Design review of the part built by this model. Coordinates are the model's own, in mm. Face numbers are marked on the shaded views. A direction names the side the tool comes from. Round coordinates to 2 decimals unless told otherwise and drop trailing zeros. Order: outer loops, then holes, each group sorted by start corner. A loop starts at its lowest first (then second) coordinate and runs counter-clockwise, first axis right, second up. Notation, with made-up numbers: (-26, -26.75) - (32, -26.75) arc R22 cw to (32, -7.75) - close; hole circle Ø11 at (21, -27.75). An arc over 180 degrees is marked (long way). Write item = value, one per line.
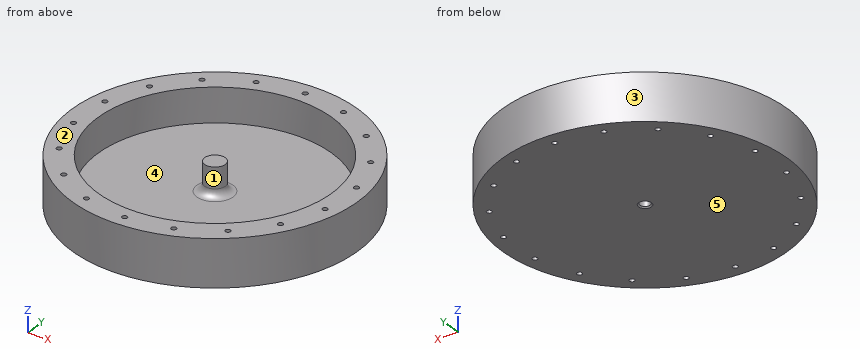
from build123d import *

# Parameters (mm, degrees)
SKETCH1_R                = 4
SKETCH1_R_2              = 2
BOSS_EXTRUDE1_DEPTH      = 8
BOSS_EXTRUDE2_START      = -8
SKETCH2_R                = 45
SKETCH2_R_2              = 4
BOSS_EXTRUDE2_DEPTH      = 5
BOSS_EXTRUDE3_START      = -8
SKETCH3_R                = 55
SKETCH3_R_2              = 45
BOSS_EXTRUDE3_DEPTH      = 18.1
SKETCH4_R                = 2
BOSS_EXTRUDE4_DEPTH      = 2
SKETCH5_R                = 1
CUT_EXTRUDE1_DEPTH       = 5
CIRPATTERN1_COUNT        = 18
MIRROR1_COPY_1_SKETCH_R  = 1
MIRROR1_COPY_1_DEPTH     = 5
MIRROR1_COPY_2_SKETCH_R  = 1
MIRROR1_COPY_2_DEPTH     = 5
MIRROR1_COPY_3_SKETCH_R  = 1
MIRROR1_COPY_3_DEPTH     = 5
MIRROR1_COPY_4_SKETCH_R  = 1
MIRROR1_COPY_4_DEPTH     = 5
MIRROR1_COPY_5_SKETCH_R  = 1
MIRROR1_COPY_5_DEPTH     = 5
MIRROR1_COPY_6_SKETCH_R  = 1
MIRROR1_COPY_6_DEPTH     = 5
MIRROR1_COPY_7_SKETCH_R  = 1
MIRROR1_COPY_7_DEPTH     = 5
MIRROR1_COPY_8_SKETCH_R  = 1
MIRROR1_COPY_8_DEPTH     = 5
MIRROR1_COPY_9_SKETCH_R  = 1
MIRROR1_COPY_9_DEPTH     = 5
MIRROR1_COPY_10_SKETCH_R = 1
MIRROR1_COPY_10_DEPTH    = 5
MIRROR1_COPY_11_SKETCH_R = 1
MIRROR1_COPY_11_DEPTH    = 5
MIRROR1_COPY_12_SKETCH_R = 1
MIRROR1_COPY_12_DEPTH    = 5
MIRROR1_COPY_13_SKETCH_R = 1
MIRROR1_COPY_13_DEPTH    = 5
MIRROR1_COPY_14_SKETCH_R = 1
MIRROR1_COPY_14_DEPTH    = 5
MIRROR1_COPY_15_SKETCH_R = 1
MIRROR1_COPY_15_DEPTH    = 5
MIRROR1_COPY_16_SKETCH_R = 1
MIRROR1_COPY_16_DEPTH    = 5
MIRROR1_COPY_17_SKETCH_R = 1
MIRROR1_COPY_17_DEPTH    = 5
CHAMFER1_SIZE            = 0.5
FILLET1_R                = 3


with BuildPart() as part:
    # Sketch1 → Boss-Extrude1 (new body, symmetric)
    with BuildSketch(Plane.XY):
        Circle(SKETCH1_R)
        Circle(SKETCH1_R_2, mode=Mode.SUBTRACT)
    extrude(amount=BOSS_EXTRUDE1_DEPTH, both=True)

    # Sketch2 → Boss-Extrude2 (add)
    with BuildSketch(Plane.XY.offset(BOSS_EXTRUDE2_START)):
        Circle(SKETCH2_R)
        Circle(SKETCH2_R_2, mode=Mode.SUBTRACT)
    extrude(amount=BOSS_EXTRUDE2_DEPTH)

    # Sketch3 → Boss-Extrude3 (add)
    with BuildSketch(Plane.XY.offset(BOSS_EXTRUDE3_START)):
        Circle(SKETCH3_R)
        Circle(SKETCH3_R_2, mode=Mode.SUBTRACT)
    extrude(amount=BOSS_EXTRUDE3_DEPTH)

    # Sketch4 → Boss-Extrude4 (add)
    with BuildSketch(Plane.XY.offset(8)):
        Circle(SKETCH4_R)
    extrude(amount=-BOSS_EXTRUDE4_DEPTH)

    # Sketch5 → Cut-Extrude1 (cut)
    with BuildSketch(Plane.XY.offset(10.1)):
        with Locations((0, 50)):
            Circle(SKETCH5_R)
    cut_extrude1 = extrude(amount=-CUT_EXTRUDE1_DEPTH, mode=Mode.SUBTRACT)

    # CirPattern1: Cut-Extrude1 ×18 about axis
    cirpattern1_axis = Axis((0, 0, 0), (0, 0, 1))
    for i in range(1, CIRPATTERN1_COUNT):
        add(cut_extrude1.rotate(cirpattern1_axis, i * 360 / CIRPATTERN1_COUNT), mode=Mode.SUBTRACT)

    # Mirror1: Cut-Extrude1 across plane
    add(cut_extrude1.mirror(Plane.XY.offset(1.05)), mode=Mode.SUBTRACT)

    # Mirror1 copy 1 sketch → Mirror1 copy 1 (cut)
    with BuildSketch(Plane(origin=(0, 0, -8), x_dir=(0.939692621, 0.342020143, 0), z_dir=(0, 0, -1))):
        with Locations((0, -50)):
            Circle(MIRROR1_COPY_1_SKETCH_R)
    extrude(amount=-MIRROR1_COPY_1_DEPTH, mode=Mode.SUBTRACT)

    # Mirror1 copy 2 sketch → Mirror1 copy 2 (cut)
    with BuildSketch(Plane(origin=(0, 0, -8), x_dir=(0.766044443, 0.64278761, 0), z_dir=(0, 0, -1))):
        with Locations((0, -50)):
            Circle(MIRROR1_COPY_2_SKETCH_R)
    extrude(amount=-MIRROR1_COPY_2_DEPTH, mode=Mode.SUBTRACT)

    # Mirror1 copy 3 sketch → Mirror1 copy 3 (cut)
    with BuildSketch(Plane(origin=(0, 0, -8), x_dir=(0.5, 0.866025404, 0), z_dir=(0, 0, -1))):
        with Locations((0, -50)):
            Circle(MIRROR1_COPY_3_SKETCH_R)
    extrude(amount=-MIRROR1_COPY_3_DEPTH, mode=Mode.SUBTRACT)

    # Mirror1 copy 4 sketch → Mirror1 copy 4 (cut)
    with BuildSketch(Plane(origin=(0, 0, -8), x_dir=(0.173648178, 0.984807753, 0), z_dir=(0, 0, -1))):
        with Locations((0, -50)):
            Circle(MIRROR1_COPY_4_SKETCH_R)
    extrude(amount=-MIRROR1_COPY_4_DEPTH, mode=Mode.SUBTRACT)

    # Mirror1 copy 5 sketch → Mirror1 copy 5 (cut)
    with BuildSketch(Plane(origin=(0, 0, -8), x_dir=(-0.173648178, 0.984807753, 0), z_dir=(0, 0, -1))):
        with Locations((0, -50)):
            Circle(MIRROR1_COPY_5_SKETCH_R)
    extrude(amount=-MIRROR1_COPY_5_DEPTH, mode=Mode.SUBTRACT)

    # Mirror1 copy 6 sketch → Mirror1 copy 6 (cut)
    with BuildSketch(Plane(origin=(0, 0, -8), x_dir=(-0.5, 0.866025404, 0), z_dir=(0, 0, -1))):
        with Locations((0, -50)):
            Circle(MIRROR1_COPY_6_SKETCH_R)
    extrude(amount=-MIRROR1_COPY_6_DEPTH, mode=Mode.SUBTRACT)

    # Mirror1 copy 7 sketch → Mirror1 copy 7 (cut)
    with BuildSketch(Plane(origin=(0, 0, -8), x_dir=(-0.766044443, 0.64278761, 0), z_dir=(0, 0, -1))):
        with Locations((0, -50)):
            Circle(MIRROR1_COPY_7_SKETCH_R)
    extrude(amount=-MIRROR1_COPY_7_DEPTH, mode=Mode.SUBTRACT)

    # Mirror1 copy 8 sketch → Mirror1 copy 8 (cut)
    with BuildSketch(Plane(origin=(0, 0, -8), x_dir=(-0.939692621, 0.342020143, 0), z_dir=(0, 0, -1))):
        with Locations((0, -50)):
            Circle(MIRROR1_COPY_8_SKETCH_R)
    extrude(amount=-MIRROR1_COPY_8_DEPTH, mode=Mode.SUBTRACT)

    # Mirror1 copy 9 sketch → Mirror1 copy 9 (cut)
    with BuildSketch(Plane(origin=(0, 0, -8), x_dir=(-1, 0, 0), z_dir=(0, 0, -1))):
        with Locations((0, -50)):
            Circle(MIRROR1_COPY_9_SKETCH_R)
    extrude(amount=-MIRROR1_COPY_9_DEPTH, mode=Mode.SUBTRACT)

    # Mirror1 copy 10 sketch → Mirror1 copy 10 (cut)
    with BuildSketch(Plane(origin=(0, 0, -8), x_dir=(-0.939692621, -0.342020143, 0), z_dir=(0, 0, -1))):
        with Locations((0, -50)):
            Circle(MIRROR1_COPY_10_SKETCH_R)
    extrude(amount=-MIRROR1_COPY_10_DEPTH, mode=Mode.SUBTRACT)

    # Mirror1 copy 11 sketch → Mirror1 copy 11 (cut)
    with BuildSketch(Plane(origin=(0, 0, -8), x_dir=(-0.766044443, -0.64278761, 0), z_dir=(0, 0, -1))):
        with Locations((0, -50)):
            Circle(MIRROR1_COPY_11_SKETCH_R)
    extrude(amount=-MIRROR1_COPY_11_DEPTH, mode=Mode.SUBTRACT)

    # Mirror1 copy 12 sketch → Mirror1 copy 12 (cut)
    with BuildSketch(Plane(origin=(0, 0, -8), x_dir=(-0.5, -0.866025404, 0), z_dir=(0, 0, -1))):
        with Locations((0, -50)):
            Circle(MIRROR1_COPY_12_SKETCH_R)
    extrude(amount=-MIRROR1_COPY_12_DEPTH, mode=Mode.SUBTRACT)

    # Mirror1 copy 13 sketch → Mirror1 copy 13 (cut)
    with BuildSketch(Plane(origin=(0, 0, -8), x_dir=(-0.173648178, -0.984807753, 0), z_dir=(0, 0, -1))):
        with Locations((0, -50)):
            Circle(MIRROR1_COPY_13_SKETCH_R)
    extrude(amount=-MIRROR1_COPY_13_DEPTH, mode=Mode.SUBTRACT)

    # Mirror1 copy 14 sketch → Mirror1 copy 14 (cut)
    with BuildSketch(Plane(origin=(0, 0, -8), x_dir=(0.173648178, -0.984807753, 0), z_dir=(0, 0, -1))):
        with Locations((0, -50)):
            Circle(MIRROR1_COPY_14_SKETCH_R)
    extrude(amount=-MIRROR1_COPY_14_DEPTH, mode=Mode.SUBTRACT)

    # Mirror1 copy 15 sketch → Mirror1 copy 15 (cut)
    with BuildSketch(Plane(origin=(0, 0, -8), x_dir=(0.5, -0.866025404, 0), z_dir=(0, 0, -1))):
        with Locations((0, -50)):
            Circle(MIRROR1_COPY_15_SKETCH_R)
    extrude(amount=-MIRROR1_COPY_15_DEPTH, mode=Mode.SUBTRACT)

    # Mirror1 copy 16 sketch → Mirror1 copy 16 (cut)
    with BuildSketch(Plane(origin=(0, 0, -8), x_dir=(0.766044443, -0.64278761, 0), z_dir=(0, 0, -1))):
        with Locations((0, -50)):
            Circle(MIRROR1_COPY_16_SKETCH_R)
    extrude(amount=-MIRROR1_COPY_16_DEPTH, mode=Mode.SUBTRACT)

    # Mirror1 copy 17 sketch → Mirror1 copy 17 (cut)
    with BuildSketch(Plane(origin=(0, 0, -8), x_dir=(0.939692621, -0.342020143, 0), z_dir=(0, 0, -1))):
        with Locations((0, -50)):
            Circle(MIRROR1_COPY_17_SKETCH_R)
    extrude(amount=-MIRROR1_COPY_17_DEPTH, mode=Mode.SUBTRACT)

    # Chamfer1
    chamfer1_edges = [part.edges().sort_by_distance(p)[0] for p in [
        (-2, 0, -8),
    ]]
    chamfer(chamfer1_edges, length=CHAMFER1_SIZE)

    # Fillet1
    fillet1_edges = [part.edges().sort_by_distance(p)[0] for p in [
        (-4, 0, -3),
    ]]
    fillet(fillet1_edges, radius=FILLET1_R)


solid = part.part
1) We need section B-B on x = -25. Write out the cut boundary in (y, z).
Findings:
outline = (-48.99, -8) - (48.99, -8) - (48.99, 10.1) - (37.42, 10.1) - (37.42, -3) - (-37.42, -3) - (-37.42, 10.1) - (-48.99, 10.1) - close
2) The part is to be moulded in two halves that separate along Y. For the marked faces 1, 2 and 3, say which applies: released by +Y, released by -Y, zero draft, split by the parting line, or undercut.
Findings:
face_1 = undercut
face_2 = zero draft
face_3 = split by the parting line
3) For the marked faces 4 and 5, list the 3-axis set-ups (+Z, -Z, +X, -X, +Y, -Y) from which the entire face can be reached by the end or side of a thin tool; tool diameter is ignored.
Findings:
face_4 = +Z
face_5 = -Z, +X, -X, +Y, -Y
4) We need section A-A on y = 0. Write out the cut boundary in (x, z), and give its area (3 significant figures).
Findings:
outline = (-55, -8) - (-2.5, -8) - (-2, -7.5) - (-2, 6) - (2, 6) - (2, -7.5) - (2.5, -8) - (55, -8) - (55, 10.1) - (45, 10.1) - (45, -3) - (7, -3) arc R3 cw to (4, 0) - (4, 8) - (-4, 8) - (-4, 0) arc R3 cw to (-7, -3) - (-45, -3) - (-45, 10.1) - (-55, 10.1) - close
area = 848 mm^2
5) We need section C-C on x = -10. Write out the cut boundary in (y, z), and give its area (3 significant figures).
Findings:
outline = (-54.08, -8) - (54.08, -8) - (54.08, 10.1) - (43.87, 10.1) - (43.87, -3) - (-43.87, -3) - (-43.87, 10.1) - (-54.08, 10.1) - close
area = 808 mm^2
6) To check wall thickness, follow L1, parallel to Y at x = 0, z = -4.5; L2, parallel to X at y = 24.5, z = -4; L3, parallel to X at y = 3, z = 6.75. State the ranges of each line that lie inside material, in increasing order. Write a range as from..to.
Findings:
L1 = -55..-51, -49..-2, 2..49, 51..55
L2 = -49.24..-44.17, -42.44..42.44, 44.17..49.24
L3 = -54.92..-44.9, -2.65..2.65, 44.9..54.92
7) Clearance check with flat-ended pins moving along their axes: pin 1 Ø1.2 at (x, y) = (-17.1, -46.98) entering from +Z; pin 2 Ø8 at (x, z) = (-18.5, 3) entering from -Y; pin 3 Ø3 at (x, y) = (-43.3, -25) entering from -Z; pin 4 Ø3 at (y, z) = (-2.5, 6) entering from +X. State where each tip first meets the part, or that it passes through.
Findings:
pin_1 = 5.1
pin_2 = -53.05
pin_3 = -8
pin_4 = 54.99
